Geometry check sheet. Reference: the model listing, model coordinates, mm. Face numbers are marked on the shaded views. A direction names the side the tool comes from. Give positions to 0.01 mm unless a question says otherwise; leave off trailing zeros. Order: outer loops, then holes, each group sorted by start corner. A loop starts at its lowest first (then second) coordinate and runs counter-clockwise, first axis right, second up. Notation, with made-up numbers: M -9,16 L 38,16 A22 ccw 38,23 Z; hole C 41,22.5 d6. An arc over 180 degrees is marked long. Put each result on its own line as item: value. Start each with the question number.
Q1. Section check B-B on y = 35. Record the cut outline in (x, z), then the cut area to 3 significant figures.
Q2. Section check D-D on y = 5. Record the cut outline in (x, z), then the cut area to 3 significant figures.
Q3. Mould release check, pull along X, two halves, no side actions. Record for the marked faces 4, 5 and 6: +X half, -X half, draft (parallel to the pull), parting line (faces both ways), or undercut.
Q4. Section check C-C on z = -39. Record the cut outline in (x, y), then the cut area to 3 significant figures.
Q5. Material ranges on L1, parallel to Y at x = -7, z = -29.5; L2, parallel to Y at x = 30, z = -14.5; L3, parallel to X at y = 42, z = -20.5, recorded low to high.
Q6. Go/stop test with flat-tipped pins: pin 1 (3 mm diameter, centred on x = 36.5, z = -8.5, fed in from -Y); pin 2 (6 mm diameter, centred on x = -11.5, z = -49, fed in from +Y); pin 3 (5 mm diameter, centred on x = 25, z = -13.5, fed in from -Y); pin 4 (1.5 mm diameter, centred on x = 30, y = 8.5, fed in from +Z). Record where each tip stops, or that it passes through.
Q7. Section check A-A on y = 16. Record the cut outline in (x, z), then the cut area to 3 significant figures.
Q8. Access from +Z, -Z, +X, -X, +Y, -Y to the whole of each face (thin tool, end or side, straight path). Record for the marked faces 1, 2 and 3.
```python
from build123d import *

# Parameters (mm, degrees)
SKETCH2_R           = 12.5
BOSS_EXTRUDE1_DEPTH = 10
BOSS_EXTRUDE2_DEPTH = 50
SKETCH5_R           = 11
CUT_EXTRUDE3_DEPTH  = 20
CUT_EXTRUDE4_DEPTH  = 20


with BuildPart() as part:
    # Sketch2 → Boss-Extrude1 (new body)
    with BuildSketch(Plane(origin=(0, 0, 0), x_dir=(1, 0, 0), z_dir=(0, 1, 0))):
        with BuildLine():
            Line((-19.074339015, 6.01411599), (0, 0))
            Line((0, 0), (19.074339015, 6.01411599))
            Line((19.074339015, 6.01411599), (16.318990173, 14.752966055))
            Line((16.318990173, 14.752966055), (29.197895289, 18.81366924))
            Line((29.197895289, 18.81366924), (19.498961292, 49.574757892))
            ThreePointArc((19.498961292, 49.574757892), (0.775540523, 64.986060166), (-19.045136415, 51.014106515))
            Line((-19.045136415, 51.014106515), (-29.197895289, 18.81366924))
            Line((-29.197895289, 18.81366924), (-16.318990173, 14.752966055))
            Line((-16.318990173, 14.752966055), (-19.074339015, 6.01411599))
        make_face()
        with Locations(Location((0.0292026, 44.999990525, 0), (0, 0, 270))):
            Circle(SKETCH2_R, mode=Mode.SUBTRACT)
    extrude(amount=BOSS_EXTRUDE1_DEPTH)

    # Sketch2_4 → Boss-Extrude2 (add)
    with BuildSketch(Plane(origin=(0, 0, 0), x_dir=(1, 0, 0), z_dir=(0, 1, 0))):
        Polygon((16.318990173, 14.752966055), (19.074339015, 6.01411599), (53.408149242, 16.839524772), (50.6528004, 25.578374837), (29.197895289, 18.81366924), align=None)
        Polygon((-53.408149242, 16.839524772), (-19.074339015, 6.01411599), (-16.318990173, 14.752966055), (-29.197895289, 18.81366924), (-50.6528004, 25.578374837), align=None)
    extrude(amount=BOSS_EXTRUDE2_DEPTH)

    # Sketch5 → Cut-Extrude3 (cut)
    with BuildSketch(Plane(origin=(0, 0, 0), x_dir=(0.9537169507482267, 0, -0.30070579950427406), z_dir=(0.300705799504274, 0, 0.9537169507482266))):
        with Locations((38, 32)):
            Circle(SKETCH5_R)
        with BuildLine():
            ThreePointArc((38, 50), (50.727922061, 44.727922061), (56, 32))
            Line((56, 32), (56, 50))
            Line((56, 50), (38, 50))
        make_face()
        with BuildLine():
            ThreePointArc((20, 32), (25.272077939, 44.727922061), (38, 50))
            Line((38, 50), (20, 50))
            Line((20, 50), (20, 32))
        make_face()
    extrude(amount=-CUT_EXTRUDE3_DEPTH, mode=Mode.SUBTRACT)

    # Sketch3 → Cut-Extrude4 (cut)
    with BuildSketch(Plane(origin=(0, 0, 0), x_dir=(0.9537169507482267, 0, 0.30070579950427406), z_dir=(-0.300705799504274, 0, 0.9537169507482266))):
        with BuildLine():
            ThreePointArc((-49, 32), (-38, 21), (-27, 32))
            Line((-27, 32), (-49, 32))
        make_face()
        with BuildLine():
            Line((-49, 32), (-27, 32))
            ThreePointArc((-27, 32), (-38, 43), (-49, 32))
        make_face()
        with BuildLine():
            ThreePointArc((-38, 50), (-25.272077939, 44.727922061), (-20, 32))
            Line((-20, 32), (-20, 50))
            Line((-20, 50), (-38, 50))
        make_face()
        with BuildLine():
            ThreePointArc((-56, 32), (-50.727922061, 44.727922061), (-38, 50))
            Line((-38, 50), (-56, 50))
            Line((-56, 50), (-56, 32))
        make_face()
    extrude(amount=-CUT_EXTRUDE4_DEPTH, mode=Mode.SUBTRACT)


solid = part.part
```
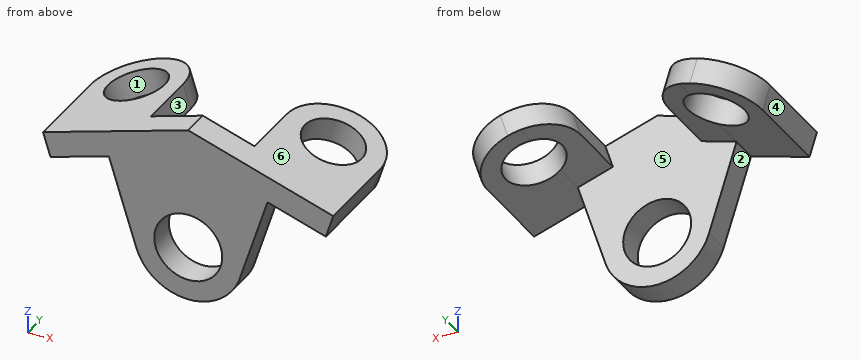
Results found:
1. outline: M -53.17,-16.76 L -50.41,-25.5 L -43.58,-23.35 L -46.33,-14.61 Z; M -26.15,-8.24 L -23.39,-16.98 L -16.56,-14.83 L -19.31,-6.09 Z; M 16.56,-14.83 L 23.39,-16.98 L 26.15,-8.24 L 19.31,-6.09 Z; M 43.58,-23.35 L 50.41,-25.5 L 53.17,-16.76 L 46.33,-14.61 Z
1. area: 263 mm^2
2. outline: M -53.41,-16.84 L -50.65,-25.58 L -29.2,-18.81 L -19.05,-51.01 A20 ccw 19.5,-49.57 L 29.2,-18.81 L 50.65,-25.58 L 53.41,-16.84 L 0,0 Z; hole C 0.03,-45 d25
2. area: 2,720 mm^2
3. face 4: -X half
3. face 5: undercut
3. face 6: +X half
4. outline: M -22.83,0 L -10.94,0 L -10.94,10 L -22.83,10 Z; M 11,0 L 22.83,0 L 22.83,10 L 11,10 Z
4. area: 237 mm^2
5. L1: y = 0 to 10
5. L2: y = 0 to 22.22, 41.78 to 49.28
5. L3: x = -49.07 to -38.19, 38.19 to 49.07
6. pin 1: passes through
6. pin 2: stops at y = 10
6. pin 3: stops at y = 0
6. pin 4: stops at z = -9.22
7. outline: M -53.41,-16.84 L -50.65,-25.58 L -16.32,-14.75 L -19.07,-6.01 Z; M 16.32,-14.75 L 50.65,-25.58 L 53.41,-16.84 L 19.07,-6.01 Z
7. area: 660 mm^2
8. face 1: none
8. face 2: -Z, +Y, -Y
8. face 3: +Z, +Y
